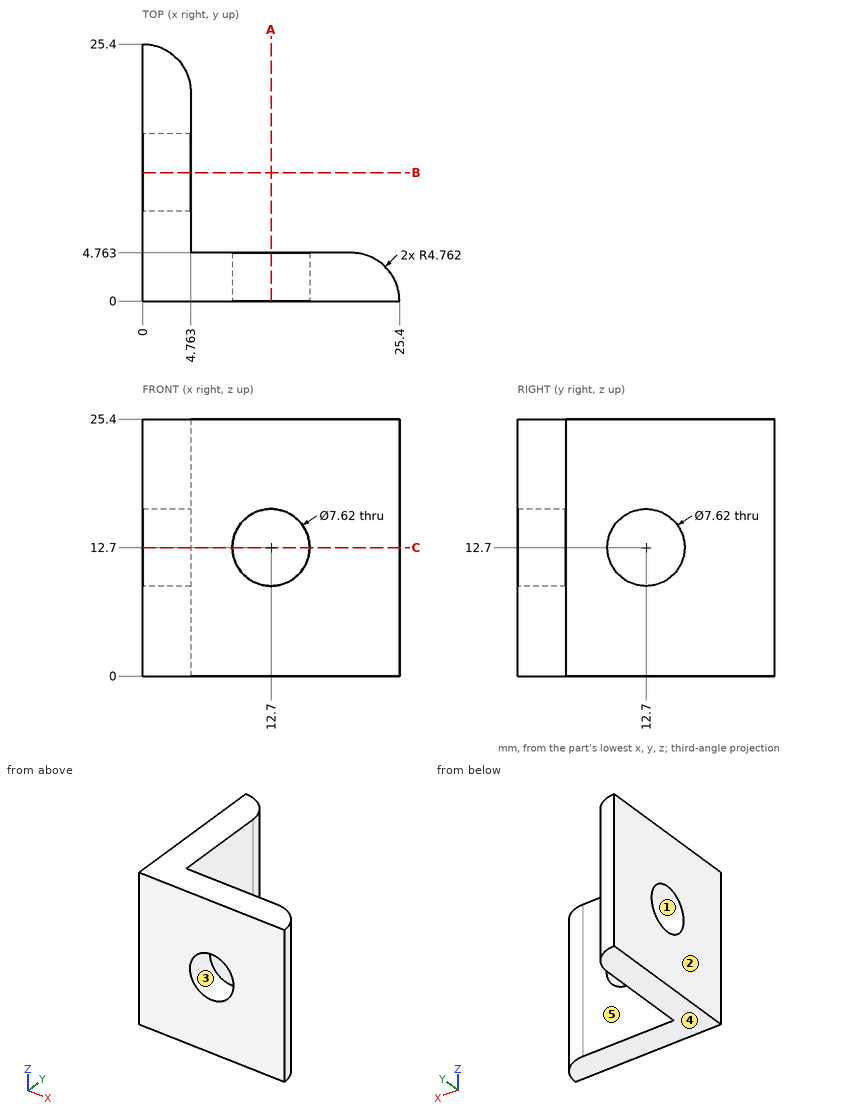
Study the drawing (mm; zero at the part's minimum x, y, z) and answer. A direction names the side the tool comes from. Round coordinates to 2 decimals unless told otherwise and drop trailing zeros. Loops run counter-clockwise (first coordinate to the right, second up) from the corner with the lowest first, then second, coordinate; pieces in that order, holes last.
Q1. Section A-A, the plane x = 12.7 is taken. Determine the outline of the cut face in (y, z).
Q2. Section C-C, the plane z = 12.7 is taken. Count the separate pieces of the cut face and the enclosed holes in it, then the cut area to 3 significant figures.
Q3. Given pin 1 Ø12 at (x, z) = (12.7, 12.7) entering from -Y; pin 2 Ø12.5 at (x, z) = (16.5, 12) entering from +Y; pin 3 Ø5 at (y, z) = (11, 9.5) entering from +X, each flat-ended and moving along its own axis, determine where each tip first touches the part or whether it passes through.
Q4. Find the intervals of material crossed by line 1 (Y direction, x = 12, z = 21.25); line 2 (Y direction, x = 3.5, z = 9.5) (1 decimal), in increasing order.
Q5. For a pull along X with two mould halves and no side action, classify the marked faces 1, 2 and 3 as released by +X, released by -X, zero draft, split by the parting line, or undercut.
Q6. Which of the six approach directions +Z, -Z, +X, -X, +Y, -Y give full straight-line access (tool end or side, diameter ignored) to the marked faces 4 and 5?
Completed:
1. outline: (0, 0) - (4.76, 0) - (4.76, 8.89) - (0, 8.89) - close; (0, 16.51) - (4.76, 16.51) - (4.76, 25.4) - (0, 25.4) - close
2. separate pieces: 3
2. enclosed holes: 0
2. area: 137 mm2
3. pin 1: stops at y = 0
3. pin 2: stops at y = 4.76
3. pin 3: stops at x = 4.76
4. line 1: y = 0 to 4.76
4. line 2: y = 0 to 10.6, 14.8 to 23.9
5. face 1: zero draft
5. face 2: released by -X
5. face 3: undercut
6. face 4: -Z, +X, -X, +Y, -Y
6. face 5: +Z, -Z, +X, +Y
